Part model, mm, in its own coordinate system. Coordinates: 2 decimals unless noted, no trailing zeros. Write each loop counter-clockwise with the first axis right and the second up, starting at its lowest first coordinate (ties: lowest second). Pieces come first, ordered by that corner, then holes. Notation, with made-up numbers: (67.25, -11.5) -> (108.25, -11.5) arc R21 ccw to (108.25, 11.5) -> close; hole circle Ø1 at (11, 44.25). An arc over 180 degrees is marked (long way). One line per question, with ' | ' between items. Start each with the question number.
Item 1: Saw through at C-C (z = 1). List the corners of the cut face in (x, y) (1 decimal).
Item 2: Pin check, flat tips, straight feed: pin 1 (1 mm diameter, centred on x = -2, y = -4.5, fed in from -Z); pin 2 (4 mm diameter, centred on x = 0, y = 0, fed in from -Z). Stop position of each tip, or through.
Item 3: Saw through at A-A (x = 0). List the corners of the cut face in (y, z).
Item 4: Saw through at D-D (x = 5.25). List the corners of the cut face in (y, z), and give its area (3 significant figures).
Item 5: Probe probe 1 along Y at (x, z) = (0, 0.5); probe 2 along X at (y, z) = (-2.5, 0.5); probe 3 along Y at (x, z) = (-1.5, 0.25). List the from-to ranges inside material, lowest first. Write a range as [from, to].
Item 6: Saw through at B-B (y = -1.25). List the corners of the cut face in (x, z).
from build123d import *

# Parameters (mm, degrees)
SKETCH1_R            = 7.9375
SKETCH1_R_2          = 3
BOSS_EXTRUDE1_DEPTH  = 1.5875
M6_CLEARANCE_HOLE1_D = 6.6


with BuildPart() as part:
    # Sketch1 → Boss-Extrude1 (new body)
    # profile 1 of 3: a face of its own
    with BuildSketch(Plane.XY):
        Circle(SKETCH1_R)
        Circle(SKETCH1_R_2, mode=Mode.SUBTRACT)
    # profile 2 of 3: a face of its own
    with BuildSketch(Plane.XY):
        with BuildLine():
            ThreePointArc((7.9375, 0), (0, -7.9375), (-7.9375, 0))
            Line((-7.9375, 0), (-7.9375, -16.51))
            Line((-7.9375, -16.51), (7.9375, -16.51))
            Line((7.9375, -16.51), (7.9375, 0))
        make_face()
    # profile 3 of 3: a face of its own
    with BuildSketch(Plane.XY):
        Circle(SKETCH1_R_2)
    extrude(amount=BOSS_EXTRUDE1_DEPTH)

    # M6 Clearance Hole1 (through all)
    with Locations(Plane.XY.offset(1.5875)):
        with Locations((0, 0)):
            Hole(M6_CLEARANCE_HOLE1_D / 2)


solid = part.part
From the geometry:
1) outline: (-7.9, -16.5) -> (7.9, -16.5) -> (7.9, 0) arc R7.9 ccw to (-7.9, 0) -> close; hole circle Ø6.6 at (0, 0)
2) pin 1: z = 0 | pin 2: through
3) outline: (-16.51, 0) -> (-3.3, 0) -> (-3.3, 1.59) -> (-16.51, 1.59) -> close; (3.3, 0) -> (7.94, 0) -> (7.94, 1.59) -> (3.3, 1.59) -> close
4) outline: (-16.51, 0) -> (5.95, 0) -> (5.95, 1.59) -> (-16.51, 1.59) -> close | area: 35.7 mm2
5) probe 1: [-16.51, -3.3], [3.3, 7.94] | probe 2: [-7.94, -2.15], [2.15, 7.94] | probe 3: [-16.51, -2.94], [2.94, 7.79]
6) outline: (-7.94, 0) -> (-3.05, 0) -> (-3.05, 1.59) -> (-7.94, 1.59) -> close; (3.05, 0) -> (7.94, 0) -> (7.94, 1.59) -> (3.05, 1.59) -> close
